Could you check a few things on this model? Use its own coordinates, in mm. Round coordinates to 2 decimals unless told otherwise and drop trailing zeros. Loops run counter-clockwise (first coordinate to the right, second up) from the corner with the lowest first, then second, coordinate; pieces in that order, holes last. Notation, with made-up numbers: (-21.75, -10) -> (11.25, -10) arc R17 cw to (11.25, 21) -> close; hole circle Ø9 at (-21, 60.25). An arc over 180 degrees is marked (long way). One line per item, written item: value.
```python
from build123d import *

# Parameters (mm, degrees)
BOSS_EXTRUDE1_DEPTH = 5
FILLET2_R           = 5
FILLET3_R           = 5
FILLET4_R           = 5
FILLET5_R           = 5
FILLET6_R           = 5
FILLET7_R           = 5
FILLET8_R           = 5
FILLET9_R           = 5
SKETCH2_R           = 1.25
SKETCH2_R_2         = 2.5
CUT_EXTRUDE1_DEPTH  = 10


with BuildPart() as part:
    # Sketch1 → Boss-Extrude1 (new body)
    with BuildSketch(Plane.XY):
        Polygon((21.15, 21.15), (41.15, 36.15), (111.15, 36.15), (111.15, -36.15), (41.15, -36.15), (21.15, -21.15), (-21.15, -21.15), (-21.15, 21.15), align=None)
    extrude(amount=BOSS_EXTRUDE1_DEPTH)

    # Fillet2
    fillet2_edges = [part.edges().sort_by_distance(p)[0] for p in [
        (-21.15, -21.15, 2.5),
    ]]
    fillet(fillet2_edges, radius=FILLET2_R)

    # Fillet3
    fillet3_edges = [part.edges().sort_by_distance(p)[0] for p in [
        (-21.15, 21.15, 2.5),
    ]]
    fillet(fillet3_edges, radius=FILLET3_R)

    # Fillet4
    fillet4_edges = [part.edges().sort_by_distance(p)[0] for p in [
        (21.15, 21.15, 2.5),
    ]]
    fillet(fillet4_edges, radius=FILLET4_R)

    # Fillet5
    fillet5_edges = [part.edges().sort_by_distance(p)[0] for p in [
        (21.15, -21.15, 2.5),
    ]]
    fillet(fillet5_edges, radius=FILLET5_R)

    # Fillet6
    fillet6_edges = [part.edges().sort_by_distance(p)[0] for p in [
        (41.15, -36.15, 2.5),
    ]]
    fillet(fillet6_edges, radius=FILLET6_R)

    # Fillet7
    fillet7_edges = [part.edges().sort_by_distance(p)[0] for p in [
        (41.15, 36.15, 2.5),
    ]]
    fillet(fillet7_edges, radius=FILLET7_R)

    # Fillet8
    fillet8_edges = [part.edges().sort_by_distance(p)[0] for p in [
        (111.15, 36.15, 2.5),
    ]]
    fillet(fillet8_edges, radius=FILLET8_R)

    # Fillet9
    fillet9_edges = [part.edges().sort_by_distance(p)[0] for p in [
        (111.15, -36.15, 2.5),
    ]]
    fillet(fillet9_edges, radius=FILLET9_R)

    # Sketch2 → Cut-Extrude1 (cut)
    with BuildSketch(Plane.XY.offset(5)):
        with Locations((-15.5, -15.5)):
            Circle(SKETCH2_R)
        with Locations((-15.5, 15.5)):
            Circle(SKETCH2_R)
        with Locations((15.5, 15.5)):
            Circle(SKETCH2_R)
        with Locations((15.5, -15.5)):
            Circle(SKETCH2_R)
        with Locations((106.15, 31.15)):
            Circle(SKETCH2_R_2)
        with Locations((106.15, -31.15)):
            Circle(SKETCH2_R_2)
        with Locations((43.95, -31.15)):
            Circle(SKETCH2_R_2)
        with Locations((43.95, 31.15)):
            Circle(SKETCH2_R_2)
        with Locations((102.55, 0)):
            Circle(SKETCH2_R_2)
        with Locations((47.55, 0)):
            Circle(SKETCH2_R_2)
    extrude(amount=-CUT_EXTRUDE1_DEPTH, mode=Mode.SUBTRACT)


solid = part.part
```
Item 1: Will these pins go through, and if not, where does the flat tip stop? pin 1 Ø1.5 at (x, z) = (2.5, 2) entering from -Y; pin 2 Ø1.5 at (x, z) = (5.5, 2) entering from +Y.
Output:
pin 1: stops at y = -21.15
pin 2: stops at y = 21.15
Item 2: If we section it at A-A on z = 1.7: Count the separate pieces of the cut face and the enclosed holes in it, plus the area to 3 significant figures.
Output:
separate pieces: 1
enclosed holes: 10
area: 7,840 mm²
Item 3: If we section it at C-C on x = 13: List the corners of the cut face in (y, z) for me.
Output:
outline: (-21.15, 0) -> (21.15, 0) -> (21.15, 5) -> (-21.15, 5) -> close
Item 4: If we section it at B-B on y = -24: List the corners of the cut face in (x, z) for me, plus the area to 3 significant figures.
Output:
outline: (24.95, 0) -> (111.15, 0) -> (111.15, 5) -> (24.95, 5) -> close
area: 431 mm²
Item 5: If we mould it in two halves opening along X, with no side actions, what happens to faces 1 (the face through (45.052, 0.11, 2.535)), 2 (the face through (1, 21.15, 2)), 3 (the face through (31.03, 28.56, 2.46))? For each: released by +X, released by -X, zero draft, split by the parting line, or undercut.
Output:
face 1: undercut
face 2: zero draft
face 3: released by -X
Item 6: I need wall thicknesses on line 1 (Y direction, x = 15.5, z = 3.15); line 2 (Y direction, x = 43.95, z = 2.5); line 3 (Y direction, x = 103.5, z = 0.45). Which ranges of each line are inside material? Lowest first, please. Write a range as from..to.
Output:
line 1: y = -21.15..-16.75, -14.25..14.25, 16.75..21.15
line 2: y = -36.15..-33.65, -28.65..28.65, 33.65..36.15
line 3: y = -36.15..-2.31, 2.31..36.15
